Source: CAD feature listing. Evaluate the final solid. Frame: model axes, mm. A direction names the side the tool comes from. Coordinates: 2 decimals unless noted, no trailing zeros. Order: outer loops, then holes, each group sorted by start corner. A loop starts at its lowest first (then second) coordinate and runs counter-clockwise, first axis right, second up.
```python
from build123d import *

# Parameters (mm, degrees)
SKETCH1_W            = 50.8
SKETCH1_H            = 50.8
SKETCH1_W_2          = 44.45
SKETCH1_H_2          = 44.45
BOSS_EXTRUDE1_DEPTH  = 76.2
SKETCH3_R            = 2.5527
CUT_EXTRUDE1_DEPTH   = 50.8
CIRPATTERN1_COUNT    = 12
SKETCH4_R            = 10.16
CUT_EXTRUDE2_DEPTH   = 50.8
SKETCH5_R            = 2.5527
CUT_EXTRUDE3_DEPTH   = 50.8
LPATTERN1_COUNT      = 3
LPATTERN1_PITCH      = 25.4
LPATTERN1_COUNT_DIR2 = 2
LPATTERN1_PITCH_DIR2 = 25.4


with BuildPart() as part:
    # Sketch1 → Boss-Extrude1 (new body)
    with BuildSketch(Plane(origin=(0, 0, 0), x_dir=(1, 0, 0), z_dir=(0, 1, 0))):
        Rectangle(SKETCH1_W, SKETCH1_H)
        Rectangle(SKETCH1_W_2, SKETCH1_H_2, mode=Mode.SUBTRACT)
    extrude(amount=BOSS_EXTRUDE1_DEPTH)

    # Sketch3 → Cut-Extrude1 (cut)
    with BuildSketch(Plane.XY.offset(25.4)):
        with Locations((0, 12.7)):
            Circle(SKETCH3_R)
    cut_extrude1 = extrude(amount=-CUT_EXTRUDE1_DEPTH, mode=Mode.SUBTRACT)

    # CirPattern1: Cut-Extrude1 ×12 about axis, 6 skipped
    cirpattern1_axis = Axis((0, 38.1, 0), (0, 0, 1))
    add([cut_extrude1.rotate(cirpattern1_axis, i * 360 / CIRPATTERN1_COUNT) for i in range(1, CIRPATTERN1_COUNT) if i not in (2, 3, 4, 8, 9, 10)], mode=Mode.SUBTRACT)

    # Sketch4 → Cut-Extrude2 (cut)
    with BuildSketch(Plane.XY.offset(25.4)):
        with Locations((0, 38.1)):
            Circle(SKETCH4_R)
    extrude(amount=-CUT_EXTRUDE2_DEPTH, mode=Mode.SUBTRACT)

    # Sketch5 → Cut-Extrude3 (cut)
    with BuildSketch(Plane.ZY.offset(25.4)):
        with Locations((-12.7, 12.7)):
            Circle(SKETCH5_R)
    cut_extrude3 = extrude(amount=-CUT_EXTRUDE3_DEPTH, mode=Mode.SUBTRACT)

    # LPattern1: Cut-Extrude3 3 × 2
    with Locations(*[(0, i * LPATTERN1_PITCH, j * LPATTERN1_PITCH_DIR2) for i in range(LPATTERN1_COUNT) for j in range(LPATTERN1_COUNT_DIR2) if (i, j) != (0, 0)]):
        add(cut_extrude3, mode=Mode.SUBTRACT)


solid = part.part
```
Q1. Set-up query: faces 3 (the flat face through (22.225, 38, 0)), 4 (the cylindrical face through (12.812, 62.647, -23.79)). Return all of +Z, -Z, +X, -X, +Y, -Y with unobstructed straight access to the full face (end or side cutting, diameter ignored); none if empty.
Solutions:
face 3: +Y, -Y
face 4: +Z, -Z
Q2. Section query C-C on x = 21. Output: boundary loops of the cut face in (y, z) (3 decimals), plus the area to 3 significant figures.
Solutions:
outline: (0, -25.4) - (76.2, -25.4) - (76.2, -22.225) - (0, -22.225) - close; (0, 22.225) - (76.2, 22.225) - (76.2, 25.4) - (0, 25.4) - close
area: 484 mm2
Q3. Section query D-D on y = 68. Output: boundary loops of the cut face in (x, z) (3 decimals).
Solutions:
outline: (-25.4, -25.4) - (25.4, -25.4) - (25.4, 25.4) - (-25.4, 25.4) - close; hole (-22.225, -22.225) - (22.225, -22.225) - (22.225, 22.225) - (-22.225, 22.225) - close
Q4. Material intervals for line 1 along X through (y, z) = (29.5, 16) (3 decimals); line 2 along Y through (x, z) = (23.45, 12.7), sorted ascending.
Solutions:
line 1: x = -25.4 to -22.225, 22.225 to 25.4
line 2: y = 0 to 10.15, 15.25 to 35.55, 40.65 to 60.95, 66.05 to 76.2
Q5. Section query B-B on z = 12.7. Give the number of separate pieces and of enclosed holes in the cut face, plus the area to 3 significant figures.
Solutions:
separate pieces: 8
enclosed holes: 0
area: 387 mm2
Q6. Pull-direction query (Y, two-part tool) for faces 1 (the cylindrical face through (-2.2, 28.18, 23.83)), 2 (the flat face through (-5, 29, 22.225)); classes: pulls with the +Y half, pulls with the -Y half, needs draft (parallel to the pull), parting line crosses it, or undercut.
Solutions:
face 1: undercut
face 2: needs draft
Q7. Section query A-A on z = -6. Output: boundary loops of the cut face in (x, y) (3 decimals), plus the area to 3 significant figures.
Solutions:
outline: (-25.4, 0) - (-22.225, 0) - (-22.225, 76.2) - (-25.4, 76.2) - close; (22.225, 0) - (25.4, 0) - (25.4, 76.2) - (22.225, 76.2) - close
area: 484 mm2
